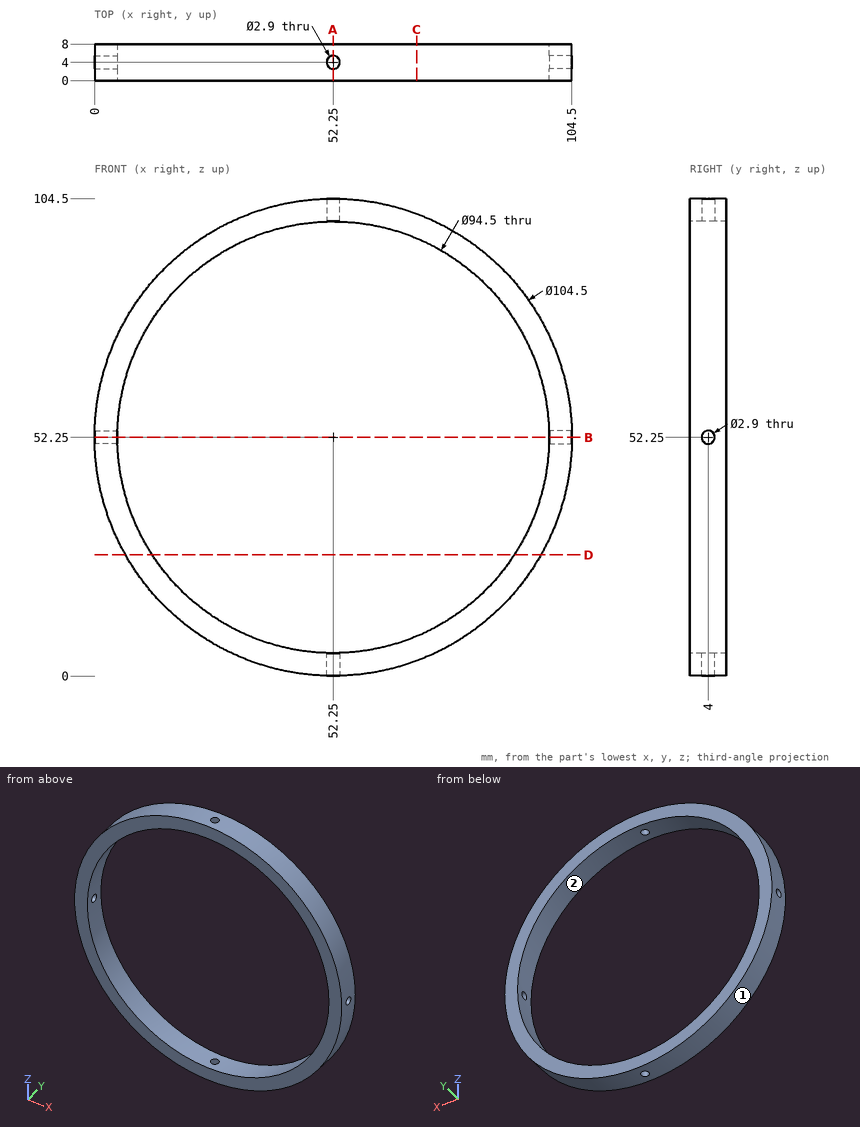
Part print with two shaded views. Sizes in mm from the minimum x, y, z corner. Round coordinates to 2 decimals unless told otherwise and drop trailing zeros. Order: outer loops, then holes, each group sorted by start corner. A loop starts at its lowest first (then second) coordinate and runs counter-clockwise, first axis right, second up. Notation, with made-up numbers: M 89,-27.5 L 102,-27.5 A19 ccw 102,-21.5 Z; hole C 76.25,9 d6. An arc over 180 degrees is marked long. Put each result on its own line as item: value. Start each with the question number.
1. Slice it at C-C on x = 70.5. List the corners of the cut face in (y, z), then the cut area to 3 significant figures.
2. Drop flat-ended pins along their axis: pin 1 (1 mm diameter, centred on x = 29.5, z = 93.5, fed in from -Y); pin 2 (2 mm diameter, centred on y = 1, z = 21.5, fed in from -X); pin 3 (2.5 mm diameter, centred on x = 52.25, y = 4, fed in from -Z); pin 4 (3 mm diameter, centred on x = 60.5, y = 3.5, fed in from -Z). Give the stop position or say it passes through.
3. Slice it at D-D on z = 26.5. List the corners of the cut face in (x, y).
4. Slice it at A-A on x = 52.25. List the corners of the cut face in (y, z).
5. Drill centre lines: probe 1 along Z at (x, y) = (52.25, 6); probe 2 along X at (y, z) = (6, 75.5); probe 3 along X at (y, z) = (3.75, 92). Where is each one in solid material? Low to high. Write a range as [from, to].
6. Two-plate mould, pull along X, no slides. Class the marked faces 1 and 2: +X half, -X half, draft (parallel to the pull), parting line (faces both ways), or undercut.
7. Slice it at B-B on z = 52.25. List the corners of the cut face in (x, y), then the cut area to 3 significant figures.
Findings:
1. outline: M 0,3.29 L 8,3.29 L 8,8.67 L 0,8.67 Z; M 0,95.83 L 8,95.83 L 8,101.21 L 0,101.21 Z
1. area: 86.0 mm2
2. pin 1: y = 0
2. pin 2: x = 9.3
2. pin 3: through
2. pin 4: z = 0.44
3. outline: M 6.79,0 L 12.63,0 L 12.63,8 L 6.79,8 Z; M 91.87,0 L 97.71,0 L 97.71,8 L 91.87,8 Z
4. outline: M 0,0 L 2.55,0 L 2.55,5 L 0,5 Z; M 0,99.5 L 2.55,99.5 L 2.55,104.5 L 0,104.5 Z; M 5.45,0 L 8,0 L 8,5 L 5.45,5 Z; M 5.45,99.5 L 8,99.5 L 8,104.5 L 5.45,104.5 Z
5. probe 1: [0, 5], [99.5, 104.5]
5. probe 2: [5.46, 11.12], [93.38, 99.04]
5. probe 3: [18.34, 26.71], [77.79, 86.16]
6. face 1: parting line
6. face 2: undercut
7. outline: M 0,0 L 5,0 L 5,2.55 L 0,2.55 Z; M 0,5.45 L 5,5.45 L 5,8 L 0,8 Z; M 99.5,0 L 104.5,0 L 104.5,2.55 L 99.5,2.55 Z; M 99.5,5.45 L 104.5,5.45 L 104.5,8 L 99.5,8 Z
7. area: 51.0 mm2
